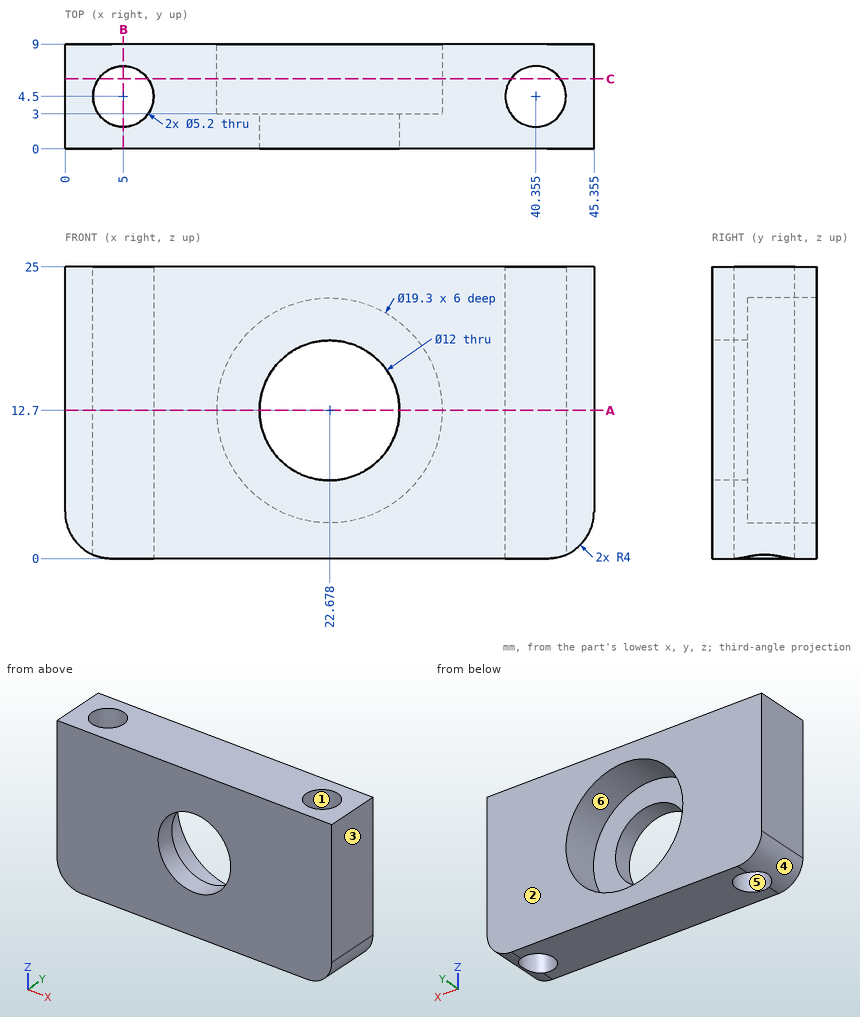
The drawing under review shows one solid part. Ordinate dimensions are in mm from its lowest x, y, z. A direction names the side the tool comes from. Give positions to 0.01 mm unless a question says otherwise; leave off trailing zeros. Loops run counter-clockwise (first coordinate to the right, second up) from the corner with the lowest first, then second, coordinate; pieces in that order, holes last. Notation, with made-up numbers: M 8.25,39.25 L 15.25,39.25 A15 ccw 15.25,57.25 Z; hole C 63.25,83.5 d1. An arc over 180 degrees is marked long. One line per item, written item: value. Start each with the question number.
Q1. For L1, parallel to X at y = 3.75, z = 4.25 (1 decimal); L2, parallel to X at y = 3.5, z = 10.75 (1 decimal); L3, parallel to X at y = 7.5, z = 15.25 (1 decimal), list the stretches that pass through material, from the lowest coordinate up.
Q2. Draft analysis for pull direction X (two halves, no side actions). For the marked faces 1, 2, 3 and 4, state which applies: released by +X, released by -X, zero draft, split by the parting line, or undercut.
Q3. Add section C-C (y = 6). Count the separate pieces of the cut face and the enclosed holes in it, and give its area (3 significant figures).
Q4. Add section B-B (x = 5). Give the boundary of the cut face in (y, z).
Q5. Add section A-A (z = 12.7). Give the boundary of the cut face in (x, y) (1 decimal), and give its area (3 significant figures).
Q6. Machinability: for the marked faces 5 and 6, which of the approach directions +Z, -Z, +X, -X, +Y, -Y give a long, thin tool a straight path to every point of the face, cutting with its end or side? Answer none if there is none.
Reply:
1. L1: 0 to 2.5, 7.5 to 18, 27.3 to 37.9, 42.8 to 45.4
1. L2: 0 to 2.6, 7.4 to 13.2, 32.1 to 38, 42.8 to 45.4
1. L3: 0 to 13.4, 32 to 45.4
2. face 1: undercut
2. face 2: zero draft
2. face 3: released by +X
2. face 4: released by -X
3. separate pieces: 3
3. enclosed holes: 1
3. area: 622 mm²
4. outline: M 0,0 L 1.9,0 L 1.9,25 L 0,25 Z; M 7.1,0 L 9,0 L 9,25 L 7.1,25 Z
5. outline: M 0,0 L 16.7,0 L 16.7,3 L 13,3 L 13,9 L 0,9 Z; M 28.7,0 L 45.4,0 L 45.4,9 L 32.3,9 L 32.3,3 L 28.7,3 Z; hole C 5,4.5 d5.2; hole C 40.4,4.5 d5.2
5. area: 214 mm²
6. face 5: +Z, -Z
6. face 6: +Y
